```python
from build123d import *

# Parameters (mm, degrees)
EXTRUSION1_DEPTH             = 14.5
ENL_V_MAT_EXTRU_1_DEPTH      = 12
ESQUISSE3_R                  = 9.5
ENL_V_MAT_EXTRU_4_DEPTH      = 28
ENL_V_MAT_EXTRU_4_DEPTH_BACK = 28


with BuildPart() as part:
    # Esquisse1 → Extrusion1 (new body, symmetric)
    with BuildSketch(Plane(origin=(0, 0, 0), x_dir=(0, 0, -1), z_dir=(1, 0, 0))):
        with BuildLine():
            Line((-27, 1), (-27, 2.85608673))
            ThreePointArc((-27, 2.85608673), (-26.840774329, 3.397472477), (-26.413802944, 3.766453207))
            Line((-26.413802944, 3.766453207), (-10.69719375, 10.910366477))
            ThreePointArc((-10.69719375, 10.910366477), (-10.495090501, 10.977334763), (-10.283390805, 11))
            Line((-10.283390805, 11), (10.283390805, 11))
            ThreePointArc((10.283390805, 11), (10.495090501, 10.977334763), (10.69719375, 10.910366477))
            Line((10.69719375, 10.910366477), (26.413802944, 3.766453207))
            ThreePointArc((26.413802944, 3.766453207), (26.840774329, 3.397472477), (27, 2.85608673))
            Line((27, 2.85608673), (27, 1))
            ThreePointArc((27, 1), (26.707106781, 0.292893219), (26, 0))
            Line((26, 0), (25.531128874, 0))
            ThreePointArc((25.531128874, 0), (25.004082597, 0.150163414), (24.635322458, 0.555555556))
            ThreePointArc((24.635322458, 0.555555556), (21.5, 2.5), (18.364677542, 0.555555556))
            ThreePointArc((18.364677542, 0.555555556), (17.995917403, 0.150163414), (17.468871126, 0))
            Line((17.468871126, 0), (-17.468871126, 0))
            ThreePointArc((-17.468871126, 0), (-17.995917403, 0.150163414), (-18.364677542, 0.555555556))
            ThreePointArc((-18.364677542, 0.555555556), (-21.5, 2.5), (-24.635322458, 0.555555556))
            ThreePointArc((-24.635322458, 0.555555556), (-25.004082597, 0.150163414), (-25.531128874, 0))
            Line((-25.531128874, 0), (-26, 0))
            ThreePointArc((-26, 0), (-26.707106781, 0.292893219), (-27, 1))
        make_face()
        with BuildLine():
            Line((-5.5, 8), (5.5, 8))
            ThreePointArc((5.5, 8), (6.207106781, 7.707106781), (6.5, 7))
            Line((6.5, 7), (6.5, 4))
            ThreePointArc((6.5, 4), (6.207106781, 3.292893219), (5.5, 3))
            Line((5.5, 3), (-5.5, 3))
            ThreePointArc((-5.5, 3), (-6.207106781, 3.292893219), (-6.5, 4))
            Line((-6.5, 4), (-6.5, 7))
            ThreePointArc((-6.5, 7), (-6.207106781, 7.707106781), (-5.5, 8))
        make_face(mode=Mode.SUBTRACT)
        with BuildLine():
            Line((-9.5, 6.606165101), (-9.5, 4))
            ThreePointArc((-9.5, 4), (-9.792893219, 3.292893219), (-10.5, 3))
            Line((-10.5, 3), (-16.233563221, 3))
            ThreePointArc((-16.233563221, 3), (-17.210897984, 3.788300304), (-16.647366165, 4.910366477))
            Line((-16.647366165, 4.910366477), (-10.913802944, 7.516531578))
            ThreePointArc((-10.913802944, 7.516531578), (-9.958614252, 7.446939429), (-9.5, 6.606165101))
        make_face(mode=Mode.SUBTRACT)
        with BuildLine():
            Line((9.5, 6.606165101), (9.5, 4))
            ThreePointArc((9.5, 4), (9.792893219, 3.292893219), (10.5, 3))
            Line((10.5, 3), (16.233563221, 3))
            ThreePointArc((16.233563221, 3), (17.210897984, 3.788300304), (16.647366165, 4.910366477))
            Line((16.647366165, 4.910366477), (10.913802944, 7.516531578))
            ThreePointArc((10.913802944, 7.516531578), (9.958614252, 7.446939429), (9.5, 6.606165101))
        make_face(mode=Mode.SUBTRACT)
    extrude(amount=EXTRUSION1_DEPTH, both=True)

    # Esquisse2 → Enlèv. mat.-Extru.1 (cut, through all)
    with BuildSketch(Plane.XZ):
        with BuildLine():
            Line((-4.75, 4.5), (4.75, 4.5))
            ThreePointArc((4.75, 4.5), (9.25, 0), (4.75, -4.5))
            Line((4.75, -4.5), (-4.75, -4.5))
            ThreePointArc((-4.75, -4.5), (-9.25, 0), (-4.75, 4.5))
        make_face()
    extrude(amount=-ENL_V_MAT_EXTRU_1_DEPTH, mode=Mode.SUBTRACT)

    # Esquisse3 → Enlèv. mat.-Extru.4 (cut, two sides)
    with BuildSketch(Plane.XY) as enl_v_mat_extru_4_sk:
        with Locations((0, 17.7)):
            Circle(ESQUISSE3_R)
    extrude(amount=ENL_V_MAT_EXTRU_4_DEPTH, mode=Mode.SUBTRACT)
    extrude(enl_v_mat_extru_4_sk.sketch, amount=-ENL_V_MAT_EXTRU_4_DEPTH_BACK, mode=Mode.SUBTRACT)


solid = part.part
```
Here's how the part is built. I have some questions about the finished solid (model axes, mm). A direction names the side the tool comes from. Coordinates: 2 decimals unless noted, no trailing zeros. Write each loop counter-clockwise with the first axis right and the second up, starting at its lowest first coordinate (ties: lowest second). Pieces come first, ordered by that corner, then holes. Notation, with made-up numbers: (28.5, -28) -> (59.5, -28) arc R16 ccw to (59.5, -7) -> close; hole circle Ø6 at (-12, 76). An arc over 180 degrees is marked (long way). Use a Markdown table: item, result. Add a question column.
(1) If we section it at D-D, the plane x = -8: State how many separate pieces and enclosed holes the cut face has, and give its area (3 significant figures).
(2) If we section it at C-C, the plane z = 15: Write out the boundary of the cut face in (x, y).
(3) If we section it at B-B, the plane y = 5.75: Write out the boundary of the cut face in (x, z).
(4) Please list where these lines run through material, in increasing order: line 1 (Z direction, x = 7, y = 2); line 2 (Z direction, x = 11.75, y = 1.75); line 3 (Z direction, x = 6.75, y = 6.5).
(5) I'm going to push flat-ended pins straight in: P1, Ø2, axis at x = -10.5, y = 7.5, coming from the +Z side; P2, Ø1.7, axis at x = -1.5, z = 14.5, coming from the +Y side; P3, Ø3.5, axis at x = -1, y = 5, coming from the +Z side. Where does each tip first touch, or does it pass through?
(6) We'd pull the mould along X, two halves only. Please class faces 1 (the flat face through (0, 5, 6.5)), 2 (the flat face through (-14.5, 2, 0)), 3 (the flat face through (0, 1, 4.5)): +X half, -X half, draft (parallel to the pull), parting line (faces both ways), or undercut.
(7) If we section it at A-A, the plane z = 0: Write out the boundary of the cut face in (x, y).
(8) For faces 4 (the flat face through (0.203, 6.195, 13.821)), 5 (the flat face through (0, 2, -27)), 6 (the cylindrical face through (-9.25, 1.48, -0.1)), which set-ups out of +Z, -Z, +X, -X, +Y, -Y let a thin tool reach every point of the face, with its end or its side?
Outcome:
| question | item | result |
|---|---|---|
| 1 | separate pieces | 2 |
| 1 | enclosed holes | 2 |
| 1 | area | 293 mm^2 |
| 2 | outline | (-14.5, 0) -> (14.5, 0) -> (14.5, 3) -> (-14.5, 3) -> close; (-14.5, 5.66) -> (14.5, 5.66) -> (14.5, 8.95) -> (3.71, 8.95) arc R9.5 cw to (-3.71, 8.95) -> (-14.5, 8.95) -> close |
| 3 | outline | (-14.5, -22.05) -> (14.5, -22.05) -> (14.5, -14.8) -> (-14.5, -14.8) -> close; (-14.5, -9.5) -> (14.5, -9.5) -> (14.5, -6.5) -> (-14.5, -6.5) -> close; (-14.5, 6.5) -> (14.5, 6.5) -> (14.5, 9.5) -> (-14.5, 9.5) -> close; (-14.5, 14.8) -> (14.5, 14.8) -> (14.5, 22.05) -> (-14.5, 22.05) -> close |
| 4 | line 1 | z = -27 to -23.3, -19.7 to -3.9, 3.9 to 19.7, 23.3 to 27 |
| 4 | line 2 | z = -27 to -23.67, -19.33 to 19.33, 23.67 to 27 |
| 4 | line 3 | z = -20.4 to -13.15, -9.5 to -6.5, 6.5 to 9.5, 13.15 to 20.4 |
| 5 | P1 | stops at z = 20.4 |
| 5 | P2 | stops at y = 8.5 |
| 5 | P3 | stops at z = 26.92 |
| 6 | face 1 | draft |
| 6 | face 2 | -X half |
| 6 | face 3 | undercut |
| 7 | outline | (-14.5, 0) -> (-9.25, 0) -> (-9.25, 3) -> (-14.5, 3) -> close; (-14.5, 8) -> (-9.25, 8) -> (-9.25, 11) -> (-14.5, 11) -> close; (9.25, 0) -> (14.5, 0) -> (14.5, 3) -> (9.25, 3) -> close; (9.25, 8) -> (14.5, 8) -> (14.5, 11) -> (9.25, 11) -> close |
| 8 | face 4 | +X, -X |
| 8 | face 5 | -Z, +X, -X, +Y, -Y |
| 8 | face 6 | +Y, -Y |
